from build123d import *

# Parameters (mm, degrees)
SKETCH1_R           = 2.5
SKETCH1_R_2         = 3.2639
SKETCH1_R_3         = 6.985
SKETCH1_R_4         = 2.159
SKETCH1_R_5         = 4.7625
SKETCH1_W           = 43.18
SKETCH1_H           = 34.798
BOSS_EXTRUDE1_DEPTH = 1.4478


with BuildPart() as part:
    # Sketch1 → Boss-Extrude1 (new body)
    with BuildSketch(Plane(origin=(0, 0, 0), x_dir=(1, 0, 0), z_dir=(0, 1, 0))):
        with BuildLine():
            Line((-58.048540962, -286.823205678), (-96.148540962, -286.823205678))
            ThreePointArc((-96.148540962, -286.823205678), (-114.109053204, -279.38371792), (-121.548540962, -261.423205678))
            Line((-121.548540962, -261.423205678), (-121.548540962, -223.323205678))
            ThreePointArc((-121.548540962, -223.323205678), (-117.828797083, -214.342949557), (-108.848540962, -210.623205678))
            Line((-108.848540962, -210.623205678), (221.351459038, -210.623205678))
            ThreePointArc((221.351459038, -210.623205678), (230.331715159, -214.342949557), (234.051459038, -223.323205678))
            Line((234.051459038, -223.323205678), (234.051459038, -261.423205678))
            ThreePointArc((234.051459038, -261.423205678), (226.611971281, -279.38371792), (208.651459038, -286.823205678))
            Line((208.651459038, -286.823205678), (170.551459038, -286.823205678))
            Line((170.551459038, -286.823205678), (170.551459038, -337.623205678))
            ThreePointArc((170.551459038, -337.623205678), (168.691587099, -342.113333738), (164.201459038, -343.973205678))
            Line((164.201459038, -343.973205678), (-51.698540962, -343.973205678))
            ThreePointArc((-51.698540962, -343.973205678), (-56.188669022, -342.113333738), (-58.048540962, -337.623205678))
            Line((-58.048540962, -337.623205678), (-58.048540962, -286.823205678))
        make_face()
        with Locations(Location((-42.808540962, -292.442955678, 0), (0, 0, 270))):
            Circle(SKETCH1_R, mode=Mode.SUBTRACT)
        with Locations(Location((-17.408540962, -292.442955678, 0), (0, 0, 90))):
            Circle(SKETCH1_R, mode=Mode.SUBTRACT)
        with Locations(Location((-17.408540962, -335.305455678, 0), (0, 0, 270))):
            Circle(SKETCH1_R, mode=Mode.SUBTRACT)
        with Locations(Location((-42.808540962, -335.305455678, 0), (0, 0, 90))):
            Circle(SKETCH1_R, mode=Mode.SUBTRACT)
        with Locations(Location((129.911459038, -292.442955678, 0), (0, 0, 270))):
            Circle(SKETCH1_R, mode=Mode.SUBTRACT)
        with Locations(Location((155.311459038, -292.442955678, 0), (0, 0, 90))):
            Circle(SKETCH1_R, mode=Mode.SUBTRACT)
        with Locations(Location((155.311459038, -335.305455678, 0), (0, 0, 270))):
            Circle(SKETCH1_R, mode=Mode.SUBTRACT)
        with Locations(Location((129.911459038, -335.305455678, 0), (0, 0, 90))):
            Circle(SKETCH1_R, mode=Mode.SUBTRACT)
        with Locations(Location((40.376459038, -313.874205678, 0), (0, 0, 270))):
            Circle(SKETCH1_R_2, mode=Mode.SUBTRACT)
        with Locations(Location((56.251459038, -313.874205678, 0), (0, 0, 270))):
            Circle(SKETCH1_R_2, mode=Mode.SUBTRACT)
        with Locations(Location((72.126459038, -313.874205678, 0), (0, 0, 270))):
            Circle(SKETCH1_R_2, mode=Mode.SUBTRACT)
        with Locations(Location((-45.348540962, -223.323205678, 0), (0, 0, 270))):
            Circle(SKETCH1_R_3, mode=Mode.SUBTRACT)
        with Locations(Location((-54.873540962, -213.798205678, 0), (0, 0, 270))):
            Circle(SKETCH1_R_4, mode=Mode.SUBTRACT)
        with Locations(Location((-35.823540962, -232.848205678, 0), (0, 0, 270))):
            Circle(SKETCH1_R_4, mode=Mode.SUBTRACT)
        with Locations(Location((8.245459038, -238.817205678, 0), (0, 0, 270))):
            Circle(SKETCH1_R_5, mode=Mode.SUBTRACT)
        with Locations(Location((148.326459038, -232.848205678, 0), (0, 0, 90))):
            Circle(SKETCH1_R_4, mode=Mode.SUBTRACT)
        with Locations(Location((157.851459038, -223.323205678, 0), (0, 0, 90))):
            Circle(SKETCH1_R_3, mode=Mode.SUBTRACT)
        with Locations(Location((167.376459038, -213.798205678, 0), (0, 0, 90))):
            Circle(SKETCH1_R_4, mode=Mode.SUBTRACT)
        with Locations(Location((-108.848540962, -223.323205678, 0), (0, 0, 270))):
            Circle(SKETCH1_R_5, mode=Mode.SUBTRACT)
        with Locations(Location((221.351459038, -223.323205678, 0), (0, 0, 270))):
            Circle(SKETCH1_R_5, mode=Mode.SUBTRACT)
        with Locations((-30.108540962, -313.874205678)):
            Rectangle(SKETCH1_W, SKETCH1_H, mode=Mode.SUBTRACT)
        with Locations((142.611459038, -313.874205678)):
            Rectangle(SKETCH1_W, SKETCH1_H, mode=Mode.SUBTRACT)
        Polygon((10.975959038, -304.36377724), (10.975959038, -297.984634115), (5.451459038, -294.795062553), (-0.073040962, -297.984634115), (-0.073040962, -304.36377724), (5.451459038, -307.553348802), align=None, mode=Mode.SUBTRACT)
        Polygon((107.051459038, -307.553348802), (101.526959038, -304.36377724), (101.526959038, -297.984634115), (107.051459038, -294.795062553), (112.575959038, -297.984634115), (112.575959038, -304.36377724), align=None, mode=Mode.SUBTRACT)
        Polygon((-90.624040962, -258.233634115), (-96.148540962, -255.044062553), (-101.673040962, -258.233634115), (-101.673040962, -264.61277724), (-96.148540962, -267.802348802), (-90.624040962, -264.61277724), align=None, mode=Mode.SUBTRACT)
        Polygon((214.175959038, -264.61277724), (208.651459038, -267.802348802), (203.126959038, -264.61277724), (203.126959038, -258.233634115), (208.651459038, -255.044062553), (214.175959038, -258.233634115), align=None, mode=Mode.SUBTRACT)
    extrude(amount=BOSS_EXTRUDE1_DEPTH)


solid = part.part
Could you check a few things on this model? Use its own coordinates, in mm. Give positions to 0.01 mm unless a question says otherwise; leave off trailing zeros. Order: outer loops, then holes, each group sorted by start corner. A loop starts at its lowest first (then second) coordinate and runs counter-clockwise, first axis right, second up. Notation, with made-up numbers: (-23.5, 21.5) -> (31.5, 21.5) arc R12 ccw to (31.5, 29.5) -> close; hole circle Ø2 at (4.25, 85). An arc over 180 degrees is marked (long way). Return JSON: item names as keys, results as strings.
1. I need wall thicknesses on line 1 (X direction, y = 1.35, z = 223.5); line 2 (X direction, y = 1.2, z = 320); line 3 (X direction, y = 1.15, z = 259.5). Which ranges of each line are inside material? Lowest first, please. Write a range as from..to.
Answer list:
{"line 1": "x = -121.55..-113.61, -104.09..-52.33, -38.37..150.87, 164.83..216.59, 226.11..234.05", "line 2": "x = -58.05..-51.7, -8.52..121.02, 164.2..170.55", "line 3": "x = -121.55..-101.67, -90.62..203.13, 214.18..234.05"}
2. For pin 1 Ø0.7 at (y, z) = (1, 302) entering from +X; pin 2 Ø0.7 at (y, z) = (1, 262) entering from -X; pin 3 Ø0.7 at (x, y) = (-71.5, 0.5) entering from +Z, each with a flat end and sliding along its axis, tell me the tip position at first contact or that it passes through.
Answer list:
{"pin 1": "stops at x = 170.55", "pin 2": "stops at x = -121.55", "pin 3": "stops at z = 286.82"}
3. Imagine slicing it at C-C on z = 275. List the corners of the cut face in (x, y) for me, then the cut area to 3 significant figures.
Answer list:
{"outline": "(-117.62, 0) -> (230.12, 0) -> (230.12, 1.45) -> (-117.62, 1.45) -> close", "area": "503 mm2"}
4. Thinking about a two-plate mould opening in X: for faces 1 (the cylindrical face through (-104.83, 0.71, 225.88)), 2 (the cylindrical face through (-113.91, 0.71, 279.58)), 3 (the cylindrical face through (226.808, 0.714, 279.185)), which applies, pulls with the +X half, pulls with the -X half, needs draft (parallel to the pull), parting line crosses it, or undercut?
Answer list:
{"face 1": "undercut", "face 2": "pulls with the -X half", "face 3": "pulls with the +X half"}
5. Imagine slicing it at B-B on y = 0.5. Give the number of separate pieces and of enclosed holes in the cut face, then the cut area to 3 significant figures.
Answer list:
{"separate pieces": "1", "enclosed holes": "26", "area": "35,500 mm2"}
6. Imagine slicing it at A-A on z = 239. List the corners of the cut face in (x, y) for me.
Answer list:
{"outline": "(-121.55, 0) -> (3.49, 0) -> (3.49, 1.45) -> (-121.55, 1.45) -> close; (13, 0) -> (234.05, 0) -> (234.05, 1.45) -> (13, 1.45) -> close"}
